Work out the finished part from the listing and answer in its coordinate system (mm). A direction names the side the tool comes from. Round coordinates to 2 decimals unless told otherwise and drop trailing zeros. Loops run counter-clockwise (first coordinate to the right, second up) from the corner with the lowest first, then second, coordinate; pieces in that order, holes last. Notation, with made-up numbers: (40, 28.25) - (44, 28.25) arc R23 cw to (44, 51.25) - close; hole circle Ø3 at (51, 63). An arc over 180 degrees is marked (long way). Answer as CSV lines item,"result". Start each with the question number.
```python
from build123d import *

# Parameters (mm, degrees)
SKETCH1_R           = 2.55
BOSS_EXTRUDE1_DEPTH = 150


with BuildPart() as part:
    # Sketch1 → Boss-Extrude1 (new body)
    with BuildSketch(Plane.XY):
        with BuildLine():
            Line((-8.5, -10), (-2.647623804, -10))
            Line((-2.647623804, -10), (-2.647623804, -8.45))
            ThreePointArc((-2.647623804, -8.45), (-2.720847109, -8.273223305), (-2.897623804, -8.2))
            Line((-2.897623804, -8.2), (-5.25, -8.2))
            ThreePointArc((-5.25, -8.2), (-5.426776695, -8.126776695), (-5.5, -7.95))
            Line((-5.5, -7.95), (-5.5, -7.053553391))
            ThreePointArc((-5.5, -7.053553391), (-5.480969883, -6.957882533), (-5.426776695, -6.876776695))
            Line((-5.426776695, -6.876776695), (-2.523223305, -3.973223305))
            ThreePointArc((-2.523223305, -3.973223305), (-2.442117467, -3.919030117), (-2.346446609, -3.9))
            Line((-2.346446609, -3.9), (2.346446609, -3.9))
            ThreePointArc((2.346446609, -3.9), (2.442117467, -3.919030117), (2.523223305, -3.973223305))
            Line((2.523223305, -3.973223305), (5.426776695, -6.876776695))
            ThreePointArc((5.426776695, -6.876776695), (5.480969883, -6.957882533), (5.5, -7.053553391))
            Line((5.5, -7.053553391), (5.5, -7.95))
            ThreePointArc((5.5, -7.95), (5.426776695, -8.126776695), (5.25, -8.2))
            Line((5.25, -8.2), (3.35, -8.2))
            ThreePointArc((3.35, -8.2), (3.173223305, -8.273223305), (3.1, -8.45))
            Line((3.1, -8.45), (3.1, -10))
            Line((3.1, -10), (8.5, -10))
            ThreePointArc((8.5, -10), (9.560660172, -9.560660172), (10, -8.5))
            Line((10, -8.5), (10, -2.647623804))
            Line((10, -2.647623804), (8.45, -2.647623804))
            ThreePointArc((8.45, -2.647623804), (8.273223305, -2.720847109), (8.2, -2.897623804))
            Line((8.2, -2.897623804), (8.2, -5.25))
            ThreePointArc((8.2, -5.25), (8.126776695, -5.426776695), (7.95, -5.5))
            Line((7.95, -5.5), (7.053553391, -5.5))
            ThreePointArc((7.053553391, -5.5), (6.957882533, -5.480969883), (6.876776695, -5.426776695))
            Line((6.876776695, -5.426776695), (3.973223305, -2.523223305))
            ThreePointArc((3.973223305, -2.523223305), (3.919030117, -2.442117467), (3.9, -2.346446609))
            Line((3.9, -2.346446609), (3.9, 2.346446609))
            ThreePointArc((3.9, 2.346446609), (3.919030117, 2.442117467), (3.973223305, 2.523223305))
            Line((3.973223305, 2.523223305), (6.876776695, 5.426776695))
            ThreePointArc((6.876776695, 5.426776695), (6.957882533, 5.480969883), (7.053553391, 5.5))
            Line((7.053553391, 5.5), (7.95, 5.5))
            ThreePointArc((7.95, 5.5), (8.126776695, 5.426776695), (8.2, 5.25))
            Line((8.2, 5.25), (8.2, 3.35))
            ThreePointArc((8.2, 3.35), (8.273223305, 3.173223305), (8.45, 3.1))
            Line((8.45, 3.1), (10, 3.1))
            Line((10, 3.1), (10, 8.5))
            ThreePointArc((10, 8.5), (9.560660172, 9.560660172), (8.5, 10))
            Line((8.5, 10), (2.647623804, 10))
            Line((2.647623804, 10), (2.647623804, 8.45))
            ThreePointArc((2.647623804, 8.45), (2.720847109, 8.273223305), (2.897623804, 8.2))
            Line((2.897623804, 8.2), (5.25, 8.2))
            ThreePointArc((5.25, 8.2), (5.426776695, 8.126776695), (5.5, 7.95))
            Line((5.5, 7.95), (5.5, 7.053553391))
            ThreePointArc((5.5, 7.053553391), (5.480969883, 6.957882533), (5.426776695, 6.876776695))
            Line((5.426776695, 6.876776695), (2.523223305, 3.973223305))
            ThreePointArc((2.523223305, 3.973223305), (2.442117467, 3.919030117), (2.346446609, 3.9))
            Line((2.346446609, 3.9), (-2.346446609, 3.9))
            ThreePointArc((-2.346446609, 3.9), (-2.442117467, 3.919030117), (-2.523223305, 3.973223305))
            Line((-2.523223305, 3.973223305), (-5.426776695, 6.876776695))
            ThreePointArc((-5.426776695, 6.876776695), (-5.480969883, 6.957882533), (-5.5, 7.053553391))
            Line((-5.5, 7.053553391), (-5.5, 7.95))
            ThreePointArc((-5.5, 7.95), (-5.426776695, 8.126776695), (-5.25, 8.2))
            Line((-5.25, 8.2), (-3.35, 8.2))
            ThreePointArc((-3.35, 8.2), (-3.173223305, 8.273223305), (-3.1, 8.45))
            Line((-3.1, 8.45), (-3.1, 10))
            Line((-3.1, 10), (-8.5, 10))
            ThreePointArc((-8.5, 10), (-9.560660172, 9.560660172), (-10, 8.5))
            Line((-10, 8.5), (-10, 2.647623804))
            Line((-10, 2.647623804), (-8.45, 2.647623804))
            ThreePointArc((-8.45, 2.647623804), (-8.273223305, 2.720847109), (-8.2, 2.897623804))
            Line((-8.2, 2.897623804), (-8.2, 5.25))
            ThreePointArc((-8.2, 5.25), (-8.126776695, 5.426776695), (-7.95, 5.5))
            Line((-7.95, 5.5), (-7.053553391, 5.5))
            ThreePointArc((-7.053553391, 5.5), (-6.957882533, 5.480969883), (-6.876776695, 5.426776695))
            Line((-6.876776695, 5.426776695), (-3.973223305, 2.523223305))
            ThreePointArc((-3.973223305, 2.523223305), (-3.919030117, 2.442117467), (-3.9, 2.346446609))
            Line((-3.9, 2.346446609), (-3.9, -2.346446609))
            ThreePointArc((-3.9, -2.346446609), (-3.919030117, -2.442117467), (-3.973223305, -2.523223305))
            Line((-3.973223305, -2.523223305), (-6.876776695, -5.426776695))
            ThreePointArc((-6.876776695, -5.426776695), (-6.957882533, -5.480969883), (-7.053553391, -5.5))
            Line((-7.053553391, -5.5), (-7.95, -5.5))
            ThreePointArc((-7.95, -5.5), (-8.126776695, -5.426776695), (-8.2, -5.25))
            Line((-8.2, -5.25), (-8.2, -3.35))
            ThreePointArc((-8.2, -3.35), (-8.273223305, -3.173223305), (-8.45, -3.1))
            Line((-8.45, -3.1), (-10, -3.1))
            Line((-10, -3.1), (-10, -8.5))
            ThreePointArc((-10, -8.5), (-9.560660172, -9.560660172), (-8.5, -10))
        make_face()
        Circle(SKETCH1_R, mode=Mode.SUBTRACT)
    extrude(amount=BOSS_EXTRUDE1_DEPTH)


solid = part.part
```
Item 1: Find the intervals of material crossed by L1, parallel to X at y = 1, z = 69; L2, parallel to Y at x = 0, z = 99.5, in increasing order.
Item 2: Section A-A, the plane y = 0 is taken. Give the vertices of the cut face in (x, z).
Item 3: Flat-ended cylindrical pins translate along their axes: pin 1 Ø2 at (x, y) = (2.5, 7.5) entering from -Z; pin 2 Ø0.8 at (y, z) = (9, 72.5) entering from -X; pin 3 Ø0.8 at (y, z) = (9.5, 104) entering from +X; pin 4 Ø0.8 at (x, z) = (-9.5, 104.5) entering from -Y. Find the tip coordinate at first contact, or state that the pin passes through.
Item 4: Determine the mould class of faces 3 (the face through (3.95, -5.4, 73.95)), 4 (the face through (-6, -10, 74)), 5 (the face through (0, 3.9, 74)) for opening direction Y: pulls with the +Y half, pulls with the -Y half, needs draft (parallel to the pull), parting line crosses it, or undercut.
Item 5: Which of the six approach directions +Z, -Z, +X, -X, +Y, -Y give full straight-line access (tool end or side, diameter ignored) to faces 1 (the face through (-2, 2, 0)), 2 (the face through (-8.2, 4, 74))?
Answer:
1,L1,"x = -3.9 to -2.35, 2.35 to 3.9"
1,L2,"y = -3.9 to -2.55, 2.55 to 3.9"
2,outline,"(-3.9, 0) - (-2.55, 0) - (-2.55, 150) - (-3.9, 150) - close; (2.55, 0) - (3.9, 0) - (3.9, 150) - (2.55, 150) - close"
3,pin 1,"stops at z = 0"
3,pin 2,"stops at x = -10"
3,pin 3,"stops at x = 9.87"
3,pin 4,"stops at y = -9.87"
4,face 3,"undercut"
4,face 4,"pulls with the -Y half"
4,face 5,"pulls with the +Y half"
5,face 1,"-Z, +X, -X, +Y, -Y"
5,face 2,"+Z, -Z"
